For this review, take the finished solid that the model builds, in its own axes (mm). A direction names the side the tool comes from. Round coordinates to 2 decimals unless told otherwise and drop trailing zeros. Order: outer loops, then holes, each group sorted by start corner. A loop starts at its lowest first (then second) coordinate and runs counter-clockwise, first axis right, second up. Notation, with made-up numbers: M 23.25,67 L 68.25,67 A16 cw 68.25,97 Z; hole C 42,49.25 d10. An arc over 180 degrees is marked long. Answer in a Markdown table with one row per item. Add a question column.
Autodesk Inventor part; units mm, degrees
ref_plane "YZ Plane" through (0, 0, 0) normal (1, 0, 0) x (0, 1, 0)
ref_plane "XZ Plane" through (0, 0, 0) normal (0, 1, 0) x (-1, 0, 0)
ref_plane "XY Plane" through (0, 0, 0) normal (0, 0, 1) x (1, 0, 0)
sketch "スケッチ1" plane through (0, 0, 0) normal (0, 0, 1) x (1, 0, 0)
  circle A0 centre (0, 0) radius 3
  dimension "d0" = 6
extrude "押し出し1" add sketch "スケッチ1" along normal blind 3
sketch "スケッチ2" plane through (0, 0, 3) normal (0, 0, 1) x (1, 0, 0)
  circle A0 centre (0, 0) radius 2.25
  dimension "d3" = 4.5
extrude "押し出し2" add sketch "スケッチ2" along normal blind 4
sketch "スケッチ3" plane through (0, 0, 0) normal (0, 0, -1) x (-1, 0, 0)
  circle A0 centre (0, 0) radius 2
  dimension "d6" = 4
extrude "押し出し3" cut sketch "スケッチ3" against normal blind 0.6
sketch "スケッチ4" plane through (0, 0, 0) normal (0, 0, -1) x (-1, 0, 0)
  circle A0 centre (0, 0) radius 1
  dimension "d9" = 2
extrude "押し出し4" cut sketch "スケッチ4" against normal through all
properties part number "RD009_ギアDS0.5-12" material "PVC、無可塑"
1. For faces 4 (the cylindrical face through (0, -1, 4)), 5 (the cylindrical face through (0.434, -1.952, 0.296)), list the 3-axis set-ups (+Z, -Z, +X, -X, +Y, -Y) from which the entire face can be reached by the end or side of a thin tool; tool diameter is ignored.
2. Consider section A-A on y = 0. Write out the cut boundary in (x, z).
3. Consider section D-D on y = 1.4. Write out the cut boundary in (x, z), plus the area to 3 significant figures.
4. Clearance check with flat-ended pins moving along their axes: pin 1 Ø1 at (y, z) = (2, 2.5) entering from -X; pin 2 Ø2.5 at (x, y) = (0, 0) entering from -Z. State where each tip first meets the part, or that it passes through.
5. The part is to be moulded in two halves that separate along Y. For faces 1 (the flat face through (-1, -1, 0.6)), 2 (the cylindrical face through (-0.29, -2.23, 4.97)), 3 (the flat face through (1, -2, 0)), say which applies: pulls with the +Y half, pulls with the -Y half, needs draft (parallel to the pull), parting line crosses it, or undercut.
6. To check wall thickness, follow probe 1 along Y at (x, z) = (0, 4.25); probe 2 along Z at (x, y) = (2.2, 0.7); probe 3 along Y at (x, z) = (-0.75, 0.5). State the ranges of each line that lie inside material, in increasing order. Write a range as [from, to].
7. Consider section C-C on z = 1.5. Write out the cut boundary in (x, y), plus the area to 3 significant figures.
Solved:
| question | item | result |
|---|---|---|
| 1 | face 4 | +Z, -Z |
| 1 | face 5 | -Z |
| 2 | outline | M -3,0 L -2,0 L -2,0.6 L -1,0.6 L -1,7 L -2.25,7 L -2.25,3 L -3,3 Z; M 1,0.6 L 2,0.6 L 2,0 L 3,0 L 3,3 L 2.25,3 L 2.25,7 L 1,7 Z |
| 3 | outline | M -2.65,0 L -1.43,0 L -1.43,0.6 L 1.43,0.6 L 1.43,0 L 2.65,0 L 2.65,3 L 1.76,3 L 1.76,7 L -1.76,7 L -1.76,3 L -2.65,3 Z |
| 3 | area | 28.3 mm^2 |
| 4 | pin 1 | stops at x = -2.6 |
| 4 | pin 2 | stops at z = 0.6 |
| 5 | face 1 | undercut |
| 5 | face 2 | parting line crosses it |
| 5 | face 3 | needs draft |
| 6 | probe 1 | y = [-2.25, -1], [1, 2.25] |
| 6 | probe 2 | z = [0, 3] |
| 6 | probe 3 | y = [-2.9, -1.85], [1.85, 2.9] |
| 7 | outline | C 0,0 d6; hole C 0,0 d2 |
| 7 | area | 25.1 mm^2 |
